Geometry check sheet. Reference: the model listing, model coordinates, mm. Face numbers are marked on the shaded views. A direction names the side the tool comes from. Give positions to 0.01 mm unless a question says otherwise; leave off trailing zeros. Loops run counter-clockwise (first coordinate to the right, second up) from the corner with the lowest first, then second, coordinate; pieces in that order, holes last.
1. Release check for a two-part mould opening along X. For the marked faces 6, 7 and 8 record: +X half, -X half, draft (parallel to the pull), parting line (faces both ways), or undercut.
2. Cross-section at B-B, the plane y = 0. Record the cut outline in (x, z), plus the area to 3 significant figures.
3. Tool access check on the marked faces 1, 2, 3, 4 and 5. Record the directions out of +Z, -Z, +X, -X, +Y, -Y that give a thin tool (end or side, any length) a straight path to the whole face; none if there is none.
4. Cross-section at D-D, the plane z = 0.2. Record the cut outline in (x, y), plus the area to 3 significant figures.
5. Material ranges on L1, parallel to X at y = 0, z = -2; L2, parallel to Y at x = -5, z = -2.2; L3, parallel to Z at x = -5.25, y = -1.75, recorded low to high.
6. Cross-section at A-A, the plane x = -5. Record the cut outline in (y, z).
7. Cross-section at C-C, the plane z = -1.8. Record the cut outline in (x, y), plus the area to 3 significant figures.
8. Go/stop test with flat-tipped pins: pin 1 Ø1.9 at (x, y) = (-5, 0) entering from -Z; pin 2 Ø0.7 at (x, z) = (-4.5, 0.5) entering from +Y; pin 3 Ø1.6 at (x, y) = (0.5, -3) entering from +Z. Record where each tip stops, or that it passes through.
from build123d import *

# Parameters (mm, degrees)
F0_W     = 19.8
F0_H     = 1.5
F1_DEPTH = 0.9
F2_W     = 19.8
F2_H     = 7.9
F3_DEPTH = 2.7
F4_R     = 1.6
F5_DEPTH = 1.2


with BuildPart() as f1:
    # F0 (on Top) → F1 (new body)
    with BuildSketch(Plane.XY):
        Rectangle(F0_W, F0_H)
    extrude(amount=F1_DEPTH)

    # F2 (on face) → F3 (join)
    with BuildSketch(Plane(origin=(0, 0, 0), x_dir=(1, 0, 0), z_dir=(0, 0, -1))):
        Rectangle(F2_W, F2_H)
    extrude(amount=F3_DEPTH)

    # F4 (on face) → F5 (cut)
    with BuildSketch(Plane(origin=(0, 0, -2.7), x_dir=(1, 0, 0), z_dir=(0, 0, -1))):
        with Locations((-5, 0)):
            Circle(F4_R)
        with Locations((5, 0)):
            Circle(F4_R)
    extrude(amount=-F5_DEPTH, mode=Mode.SUBTRACT)


solid = f1.part
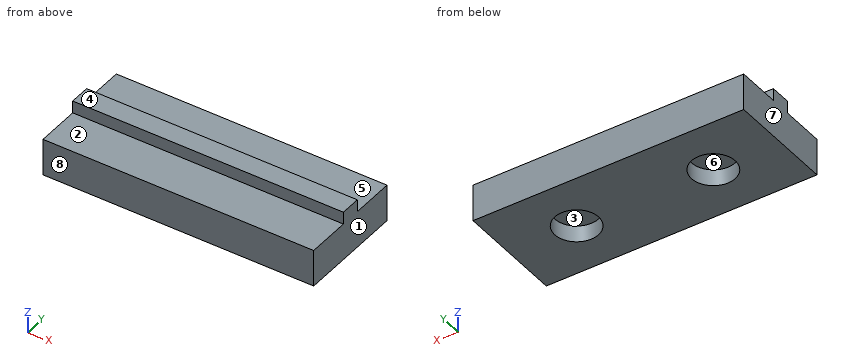
Result:
1. face 6: undercut
1. face 7: -X half
1. face 8: draft
2. outline: (-9.9, -2.7) - (-6.6, -2.7) - (-6.6, -1.5) - (-3.4, -1.5) - (-3.4, -2.7) - (3.4, -2.7) - (3.4, -1.5) - (6.6, -1.5) - (6.6, -2.7) - (9.9, -2.7) - (9.9, 0.9) - (-9.9, 0.9) - close
2. area: 63.6 mm2
3. face 1: +Z, -Z, +X, +Y, -Y
3. face 2: +Z, +X, -X, -Y
3. face 3: -Z
3. face 4: +Z, +X, -X, +Y, -Y
3. face 5: +Z, +X, -X, +Y
4. outline: (-9.9, -0.75) - (9.9, -0.75) - (9.9, 0.75) - (-9.9, 0.75) - close
4. area: 29.7 mm2
5. L1: x = -9.9 to -6.6, -3.4 to 3.4, 6.6 to 9.9
5. L2: y = -3.95 to -1.6, 1.6 to 3.95
5. L3: z = -2.7 to 0
6. outline: (-3.95, -2.7) - (-1.6, -2.7) - (-1.6, -1.5) - (1.6, -1.5) - (1.6, -2.7) - (3.95, -2.7) - (3.95, 0) - (0.75, 0) - (0.75, 0.9) - (-0.75, 0.9) - (-0.75, 0) - (-3.95, 0) - close
7. outline: (-9.9, -3.95) - (9.9, -3.95) - (9.9, 3.95) - (-9.9, 3.95) - close; hole circle Ø3.2 at (-5, 0); hole circle Ø3.2 at (5, 0)
7. area: 140 mm2
8. pin 1: stops at z = -1.5
8. pin 2: stops at y = 0.75
8. pin 3: stops at z = 0
